Source: CAD feature listing. Evaluate the final solid. Frame: model axes, mm. A direction names the side the tool comes from. Coordinates: 2 decimals unless noted, no trailing zeros. Order: outer loops, then holes, each group sorted by start corner. A loop starts at its lowest first (then second) coordinate and runs counter-clockwise, first axis right, second up. Notation, with made-up numbers: (-28, 50.5) -> (3, 50.5) arc R15 ccw to (3, 54.5) -> close; hole circle Ø3 at (54.5, 65). An arc over 180 degrees is marked (long way). Put each result on its own line as item: value.
from build123d import *

# Parameters (mm, degrees)
SKETCH1_R           = 69
BOSS_EXTRUDE1_DEPTH = 3
SKETCH2_R           = 32
BOSS_EXTRUDE2_DEPTH = 18
SKETCH3_R           = 11.7
SKETCH3_R_2         = 1.5
CUT_EXTRUDE1_DEPTH  = 22
SKETCH6_R           = 30
CUT_EXTRUDE3_DEPTH  = 18
SKETCH7_R           = 1.5
CUT_EXTRUDE5_DEPTH  = 4
SKETCH8_R           = 4.05
CUT_EXTRUDE6_DEPTH  = 1.5


with BuildPart() as part:
    # Sketch1 → Boss-Extrude1 (new body)
    with BuildSketch(Plane(origin=(0, 0, 0), x_dir=(1, 0, 0), z_dir=(0, 1, 0))):
        Circle(SKETCH1_R)
    extrude(amount=BOSS_EXTRUDE1_DEPTH)

    # Sketch2 → Boss-Extrude2 (add)
    with BuildSketch(Plane(origin=(0, 3, 0), x_dir=(1, 0, 0), z_dir=(0, 1, 0))):
        Circle(SKETCH2_R)
    extrude(amount=BOSS_EXTRUDE2_DEPTH)

    # Sketch3 → Cut-Extrude1 (cut, through all)
    with BuildSketch(Plane(origin=(0, 21, 0), x_dir=(1, 0, 0), z_dir=(0, 1, 0))):
        Circle(SKETCH3_R)
        with Locations((15.5, 15.5)):
            Circle(SKETCH3_R_2)
        with Locations((-15.5, 15.5)):
            Circle(SKETCH3_R_2)
        with Locations((15.5, -15.5)):
            Circle(SKETCH3_R_2)
        with Locations((-15.5, -15.5)):
            Circle(SKETCH3_R_2)
    extrude(amount=-CUT_EXTRUDE1_DEPTH, mode=Mode.SUBTRACT)

    # Sketch6 → Cut-Extrude3 (cut)
    with BuildSketch(Plane(origin=(0, 0, 0), x_dir=(-1, 0, 0), z_dir=(0, -1, 0))):
        Circle(SKETCH6_R)
    extrude(amount=-CUT_EXTRUDE3_DEPTH, mode=Mode.SUBTRACT)

    # Sketch7 → Cut-Extrude5 (cut, through all)
    with BuildSketch(Plane(origin=(0, 3, 0), x_dir=(1, 0, 0), z_dir=(0, 1, 0))):
        with Locations((43.133513652, 43.133513652)):
            Circle(SKETCH7_R)
        with Locations((43.133513652, -43.133513652)):
            Circle(SKETCH7_R)
        with Locations((-43.133513652, -43.133513652)):
            Circle(SKETCH7_R)
        with Locations((-43.133513652, 43.133513652)):
            Circle(SKETCH7_R)
        with BuildLine():
            Line((34.648232278, 34.648232278), (37.476659403, 37.476659403))
            ThreePointArc((37.476659403, 37.476659403), (53, 0), (37.476659403, -37.476659403))
            Line((37.476659403, -37.476659403), (34.648232278, -34.648232278))
            ThreePointArc((34.648232278, -34.648232278), (49, 0), (34.648232278, 34.648232278))
        make_face()
        with BuildLine():
            Line((-37.476659403, -37.476659403), (-34.648232278, -34.648232278))
            ThreePointArc((-34.648232278, -34.648232278), (-49, 0), (-34.648232278, 34.648232278))
            Line((-34.648232278, 34.648232278), (-37.476659403, 37.476659403))
            ThreePointArc((-37.476659403, 37.476659403), (-53, 0), (-37.476659403, -37.476659403))
        make_face()
    extrude(amount=-CUT_EXTRUDE5_DEPTH, mode=Mode.SUBTRACT)

    # Sketch8 → Cut-Extrude6 (cut)
    with BuildSketch(Plane.XZ):
        with Locations((-43.133513652, 43.133513652)):
            Circle(SKETCH8_R)
        with Locations((43.133513652, 43.133513652)):
            Circle(SKETCH8_R)
        with Locations((43.133513652, -43.133513652)):
            Circle(SKETCH8_R)
        with Locations((-43.133513652, -43.133513652)):
            Circle(SKETCH8_R)
    extrude(amount=-CUT_EXTRUDE6_DEPTH, mode=Mode.SUBTRACT)


solid = part.part
1. Cut plane C-C on z = -21.5. Output: boundary loops of the cut face in (x, y).
Numbers:
outline: (-65.56, 0) -> (-48.44, 0) -> (-48.44, 3) -> (-65.56, 3) -> close; (-44.03, 0) -> (-20.92, 0) -> (-20.92, 18) -> (20.92, 18) -> (20.92, 0) -> (44.03, 0) -> (44.03, 3) -> (23.7, 3) -> (23.7, 21) -> (-23.7, 21) -> (-23.7, 3) -> (-44.03, 3) -> close; (48.44, 0) -> (65.56, 0) -> (65.56, 3) -> (48.44, 3) -> close
2. Pull-direction query (Z, two-part tool) for faces 1 (the cylindrical face through (-44.011, 0.74, -47.087)), 2 (the flat face through (30, 0, 14)), 3 (the cylindrical face through (-6.94, 11.87, 31.24)); classes: pulls with the +Z half, pulls with the -Z half, needs draft (parallel to the pull), parting line crosses it, or undercut.
Numbers:
face 1: undercut
face 2: needs draft
face 3: parting line crosses it
3. First-contact query: pin 1 (9.5 mm diameter, centred on x = 43.13, z = -43.13, fed in from +Y); pin 2 (4 mm diameter, centred on x = 40.5, y = 4, fed in from +Z); pin 3 (6.5 mm diameter, centred on x = 43.5, z = 42.5, fed in from -Y). Flat tips, straight axial feed; report the tip coordinate or a pass-through.
Numbers:
pin 1: stops at y = 3
pin 2: stops at z = 57.08
pin 3: stops at y = 1.5
4. Set-up query: faces 4 (the cylindrical face through (-44.01, 0.74, 39.18)), 5 (the flat face through (14, 21, 0)), 6 (the cylindrical face through (-52.997, 1.521, -0.583)). Return all of +Z, -Z, +X, -X, +Y, -Y with unobstructed straight access to the full face (end or side cutting, diameter ignored); none if empty.
Numbers:
face 4: -Y
face 5: +Z, -Z, +X, -X, +Y
face 6: +Y, -Y
5. Cut plane B-B on x = 0. Output: boundary loops of the cut face in (y, z).
Numbers:
outline: (0, -69) -> (3, -69) -> (3, -32) -> (21, -32) -> (21, -11.7) -> (18, -11.7) -> (18, -30) -> (0, -30) -> close; (0, 30) -> (18, 30) -> (18, 11.7) -> (21, 11.7) -> (21, 32) -> (3, 32) -> (3, 69) -> (0, 69) -> close
6. Ray query, line 1 along X through (y, z) = (2.75, -1); line 2 along X through (y, z) = (20.25, 15.5). Return the intervals inside material, ascending.
Numbers:
line 1: x = -68.99 to -52.99, -48.99 to -29.98, 29.98 to 48.99, 52.99 to 68.99
line 2: x = -28 to -17, -14 to 14, 17 to 28
7. Cut plane A-A on z = 0. Output: boundary loops of the cut face in (x, y), plus the area to 3 significant figures.
Numbers:
outline: (-69, 0) -> (-53, 0) -> (-53, 3) -> (-69, 3) -> close; (-49, 0) -> (-30, 0) -> (-30, 18) -> (-11.7, 18) -> (-11.7, 21) -> (-32, 21) -> (-32, 3) -> (-49, 3) -> close; (11.7, 18) -> (30, 18) -> (30, 0) -> (49, 0) -> (49, 3) -> (32, 3) -> (32, 21) -> (11.7, 21) -> close; (53, 0) -> (69, 0) -> (69, 3) -> (53, 3) -> close
area: 392 mm2
8. Cut plane D-D on y = 6.5. Output: boundary loops of the cut face in (x, z).
Numbers:
outline: circle Ø64 at (0, 0); hole circle Ø60 at (0, 0)
